Input: dimensioned drawing with shaded views. Units: mm. Origin: part minimum x, y, z. Round coordinates to 2 decimals unless told otherwise and drop trailing zeros. Loops run counter-clockwise (first coordinate to the right, second up) from the corner with the lowest first, then second, coordinate; pieces in that order, holes last. Notation, with made-up numbers: (54, 47) - (112, 47) arc R16 ccw to (112, 52) - close; hole circle Ø2 at (77, 89.25). An arc over 180 degrees is marked (long way). One line per question, with ' | ' between items. Start each with the question number.
Item 1: Section A-A, the plane z = 14. Return loops of the section in (x, y), plus the area to 3 significant figures.
Item 2: Draft query along X for the marked faces 1, 2, 3 and 4. Return one class per face: pulls with the +X half, pulls with the -X half, needs draft (parallel to the pull), parting line crosses it, or undercut.
Item 3: Section D-D, the plane x = 2. Return loops of the section in (y, z) (1 decimal).
Item 4: Section B-B, the plane y = 13.97. Return loops of the section in (x, z).
Item 5: First-contact query: pin 1 (4 mm diameter, centred on y = 6.5, z = 28.5, fed in from +X); pin 2 (2 mm diameter, centred on x = 5.5, z = 1, fed in from +Y); pin 3 (1.2 mm diameter, centred on x = 5.5, z = 1, fed in from -Y). Flat tips, straight axial feed; report the tip coordinate or a pass-through.
Item 6: Material intervals for line 1 along X through (y, z) = (18.5, 18); line 2 along Y through (x, z) = (13.7, 20); line 3 along Z through (x, y) = (7.75, 12.25), sorted ascending.
Item 7: Section C-C, the plane z = 20. Return loops of the section in (x, y).
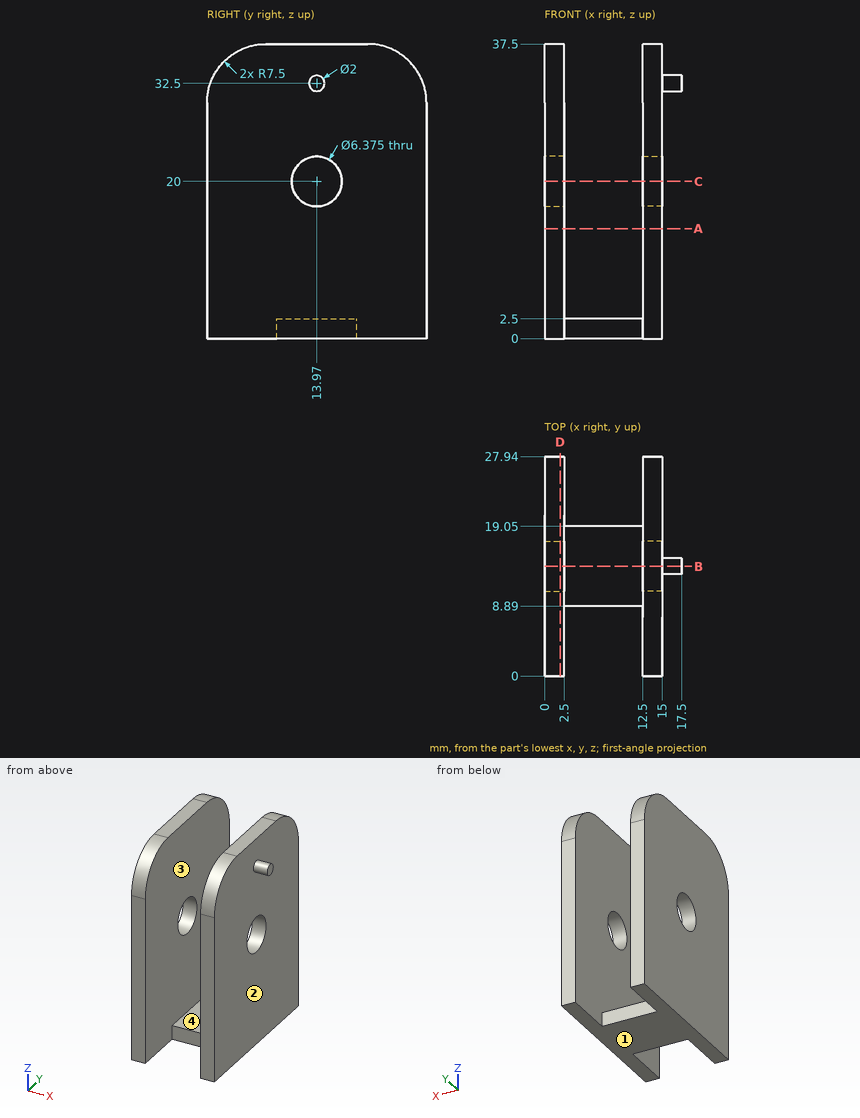
Return value:
1) outline: (0, 0) - (2.5, 0) - (2.5, 27.94) - (0, 27.94) - close; (12.5, 0) - (15, 0) - (15, 27.94) - (12.5, 27.94) - close | area: 140 mm2
2) face 1: needs draft | face 2: pulls with the +X half | face 3: undercut | face 4: undercut
3) outline: (0, 0) - (27.9, 0) - (27.9, 30) arc R7.5 ccw to (20.4, 37.5) - (7.5, 37.5) arc R7.5 ccw to (0, 30) - close; hole circle Ø6.4 at (14, 20)
4) outline: (0, 0) - (15, 0) - (15, 16.81) - (12.5, 16.81) - (12.5, 2.5) - (2.5, 2.5) - (2.5, 16.81) - (0, 16.81) - close; (0, 23.19) - (2.5, 23.19) - (2.5, 37.5) - (0, 37.5) - close; (12.5, 23.19) - (15, 23.19) - (15, 31.5) - (17.5, 31.5) - (17.5, 33.5) - (15, 33.5) - (15, 37.5) - (12.5, 37.5) - close
5) pin 1: x = 15 | pin 2: y = 19.05 | pin 3: y = 8.89
6) line 1: 0 to 2.5, 12.5 to 15 | line 2: 0 to 10.78, 17.16 to 27.94 | line 3: 0 to 2.5
7) outline: (0, 0) - (2.5, 0) - (2.5, 10.78) - (0, 10.78) - close; (0, 17.16) - (2.5, 17.16) - (2.5, 27.94) - (0, 27.94) - close; (12.5, 0) - (15, 0) - (15, 10.78) - (12.5, 10.78) - close; (12.5, 17.16) - (15, 17.16) - (15, 27.94) - (12.5, 27.94) - close
